Here's how the part is built. I have some questions about the finished solid (model axes, mm). A direction names the side the tool comes from. Round coordinates to 2 decimals unless told otherwise and drop trailing zeros. Loops run counter-clockwise (first coordinate to the right, second up) from the corner with the lowest first, then second, coordinate; pieces in that order, holes last. Notation, with made-up numbers: M 34,54.5 L 77,54.5 A16 cw 77,65.5 Z; hole C 21,21 d4. An arc over 180 degrees is marked long. Answer as CSV lines item,"result".
```python
from build123d import *

# Parameters (mm, degrees)
SKETCH_1_R               = 12.5
EXTRUDE_1_DEPTH          = 7.5
EXTRUDE_2_DEPTH          = 10
EXTRUDE_START            = -4.5
SKETCH_3_R               = 18
SKETCH_3_R_2             = 12.5
EXTRUDE_3_DEPTH          = 4.5
SKETCH_4_R               = 2.1
CUT_EXTRUDE_1_DEPTH      = 39.055354
SKETCH_5_R               = 1.6
CUT_EXTRUDE_2_DEPTH      = 39.055354
CUT_EXTRUDE_START        = -10
CUT_EXTRUDE_3_DEPTH      = 10
SKETCH_7_R               = 21
EXTRUDE_4_DEPTH          = 3
SKETCH_8_R               = 1.6
CUT_EXTRUDE_4_DEPTH      = 41.816663
SKETCH_13_R              = 15
SKETCH_13_R_2            = 12.5
EXTRUDE_6_DEPTH          = 10.5
CUT_EXTRUDE_6_DEPTH      = 39.820098
CUT_EXTRUDE_6_DEPTH_BACK = 39.820098
CUT_EXTRUDE_START_2      = 10.5
SKETCH_9_R               = 3.4
CUT_EXTRUDE_5_DEPTH      = 15
EXTRUDE_5_DEPTH          = 10
SKETCH_12_R              = 1.6
CUT_EXTRUDE_7_DEPTH      = 47.859471


# Read off the part's stored shape, not the designer's step: 凸台-拉伸2
with BuildPart() as part:
    # 草图1 → 凸台-拉伸1 (new, symmetric)
    with BuildSketch(Plane(origin=(0, 0, 0), x_dir=(1, 0, 0), z_dir=(0, 1, 0))):
        with Locations(Location((0, 0, 0), (0, 0, 270))):
            Circle(SKETCH_1_R)
        with BuildLine():
            Line((6.6, -7.6), (-6.6, -7.6))
            ThreePointArc((-6.6, -7.6), (-8.307107, -8.307107), (-7.6, -6.6))
            Line((-7.6, -6.6), (-7.6, 6.6))
            ThreePointArc((-7.6, 6.6), (-8.307107, 8.307107), (-6.6, 7.6))
            Line((-6.6, 7.6), (6.6, 7.6))
            ThreePointArc((6.6, 7.6), (7.6, 8.6), (8.6, 7.6))
            ThreePointArc((8.6, 7.6), (8.307107, 6.892893), (7.6, 6.6))
            Line((7.6, 6.6), (7.6, -6.6))
            ThreePointArc((7.6, -6.6), (8.307107, -6.892893), (8.6, -7.6))
            ThreePointArc((8.6, -7.6), (7.6, -8.6), (6.6, -7.6))
        make_face(mode=Mode.SUBTRACT)
    extrude(amount=EXTRUDE_1_DEPTH, both=True)

    # 凸台-拉伸2 outline → 凸台-拉伸2 (add)
    with BuildSketch(Plane.XZ.offset(7.5)):
        with BuildLine():
            Line((10.6, -6.624953), (10.6, 6.624953))
            ThreePointArc((10.6, 6.624953), (8.838835, 8.838835), (6.624953, 10.6))
            Line((6.624953, 10.6), (-6.624953, 10.6))
            ThreePointArc((-6.624953, 10.6), (-8.838835, 8.838835), (-10.6, 6.624953))
            Line((-10.6, 6.624953), (-10.6, -6.624953))
            ThreePointArc((-10.6, -6.624953), (-8.838835, -8.838835), (-6.624953, -10.6))
            Line((-6.624953, -10.6), (6.624953, -10.6))
            ThreePointArc((6.624953, -10.6), (8.838835, -8.838835), (10.6, -6.624953))
        make_face()
        with BuildLine():
            ThreePointArc((-6.6, -7.6), (-8.307107, -8.307107), (-7.6, -6.6))
            Line((-7.6, -6.6), (-7.6, 6.6))
            ThreePointArc((-7.6, 6.6), (-8.307107, 8.307107), (-6.6, 7.6))
            Line((-6.6, 7.6), (6.6, 7.6))
            ThreePointArc((6.6, 7.6), (8.307107, 8.307107), (7.6, 6.6))
            Line((7.6, 6.6), (7.6, -6.6))
            ThreePointArc((7.6, -6.6), (8.307107, -8.307107), (6.6, -7.6))
            Line((6.6, -7.6), (-6.6, -7.6))
        make_face(mode=Mode.SUBTRACT)
    extrude_2 = extrude(amount=EXTRUDE_2_DEPTH)

    # 镜向1: 凸台-拉伸2 across plane
    add(extrude_2.mirror(Plane.ZX))

    # 草图3 → 凸台-拉伸3 (add)
    with BuildSketch(Plane.XZ.offset(7.5).offset(EXTRUDE_START)):
        with Locations(Location((0, 0, 0), (0, 0, 270))):
            Circle(SKETCH_3_R)
        with Locations(Location((0, 0, 0), (0, 0, 270))):
            Circle(SKETCH_3_R_2, mode=Mode.SUBTRACT)
    extrude(amount=EXTRUDE_3_DEPTH)

    # 草图4 → 切除-拉伸1 (cut, through all)
    with BuildSketch(Plane.XY.offset(10.6)):
        with Locations((0, -12.5)):
            Circle(SKETCH_4_R)
    extrude(amount=-CUT_EXTRUDE_1_DEPTH, mode=Mode.SUBTRACT)

    # 草图5 → 切除-拉伸2 (cut, through all)
    with BuildSketch(Plane(origin=(10.6, 0, 0), x_dir=(0, 0, -1), z_dir=(1, 0, 0))):
        with Locations((0, 12.5)):
            Circle(SKETCH_5_R)
    extrude(amount=-CUT_EXTRUDE_2_DEPTH, mode=Mode.SUBTRACT)

    # 草图6 → 切除-拉伸3 (cut)
    with BuildSketch(Plane.XZ.offset(17.5).offset(CUT_EXTRUDE_START)):
        with BuildLine():
            Line((10.6, -6.624953), (10.6, 6.624953))
            ThreePointArc((10.6, 6.624953), (8.838835, 8.838835), (6.624953, 10.6))
            Line((6.624953, 10.6), (-6.624953, 10.6))
            ThreePointArc((-6.624953, 10.6), (-8.838835, 8.838835), (-10.6, 6.624953))
            Line((-10.6, 6.624953), (-10.6, -6.624953))
            ThreePointArc((-10.6, -6.624953), (-8.838835, -8.838835), (-6.624953, -10.6))
            Line((-6.624953, -10.6), (6.624953, -10.6))
            ThreePointArc((6.624953, -10.6), (8.838835, -8.838835), (10.6, -6.624953))
        make_face()
    extrude(amount=CUT_EXTRUDE_3_DEPTH, mode=Mode.SUBTRACT)

    # 草图7 → 凸台-拉伸4 (add)
    with BuildSketch(Plane.XZ.offset(7.5)):
        with Locations(Location((0, 0, 0), (0, 0, 270))):
            Circle(SKETCH_7_R)
    extrude(amount=EXTRUDE_4_DEPTH)

    # 草图8 → 切除-拉伸4 (cut, through all)
    with BuildSketch(Plane.XZ.offset(10.5)):
        with Locations(Location((0, 16, 0), (0, 0, 270))):
            Circle(SKETCH_8_R)
        with Locations(Location((16, 0, 0), (0, 0, 270))):
            Circle(SKETCH_8_R)
        with Locations(Location((0, -16, 0), (0, 0, 270))):
            Circle(SKETCH_8_R)
        with Locations(Location((-16, 0, 0), (0, 0, 270))):
            Circle(SKETCH_8_R)
    extrude(amount=-CUT_EXTRUDE_4_DEPTH, mode=Mode.SUBTRACT)

    # 草图13 → 凸台-拉伸6 (add)
    with BuildSketch(Plane(origin=(0, -3, 0), x_dir=(1, 0, 0), z_dir=(0, 1, 0))):
        with Locations(Location((0, 0, 0), (0, 0, 85.379415))):
            Circle(SKETCH_13_R)
        Circle(SKETCH_13_R_2, mode=Mode.SUBTRACT)
    extrude(amount=EXTRUDE_6_DEPTH)

    # 草图10 → 切除-拉伸6 (cut, two sides: drawn at the far end of the back side and taken through both)
    with BuildSketch(Plane(origin=(0, -7.5, 0), x_dir=(1, 0, 0), z_dir=(0, 1, 0)).offset(-CUT_EXTRUDE_6_DEPTH_BACK)):
        with BuildLine():
            Line((-7.6, 6.6), (-7.6, -6.6))
            ThreePointArc((-7.6, -6.6), (-8.307107, -8.307107), (-6.6, -7.6))
            Line((-6.6, -7.6), (6.6, -7.6))
            ThreePointArc((6.6, -7.6), (8.307107, -8.307107), (7.6, -6.6))
            Line((7.6, -6.6), (7.6, 6.6))
            ThreePointArc((7.6, 6.6), (8.307107, 8.307107), (6.6, 7.6))
            Line((6.6, 7.6), (-6.6, 7.6))
            ThreePointArc((-6.6, 7.6), (-8.307107, 8.307107), (-7.6, 6.6))
        make_face()
    extrude(amount=CUT_EXTRUDE_6_DEPTH + CUT_EXTRUDE_6_DEPTH_BACK, mode=Mode.SUBTRACT)

    # 草图9 → 切除-拉伸5 (cut)
    with BuildSketch(Plane(origin=(0, -3, 0), x_dir=(1, 0, 0), z_dir=(0, 1, 0)).offset(CUT_EXTRUDE_START_2)):
        with Locations((0, -16)):
            Circle(SKETCH_9_R)
        with Locations((16, 0)):
            Circle(SKETCH_9_R)
        with Locations((0, 16)):
            Circle(SKETCH_9_R)
        with Locations((-16, 0)):
            Circle(SKETCH_9_R)
    extrude(amount=-CUT_EXTRUDE_5_DEPTH, mode=Mode.SUBTRACT)

    # 草图11 → 凸台-拉伸5 (add)
    with BuildSketch(Plane(origin=(0, 17.5, 0), x_dir=(1, 0, 0), z_dir=(0, 1, 0))):
        with BuildLine():
            Line((6.624953, 10.6), (-6.624953, 10.6))
            ThreePointArc((-6.624953, 10.6), (-8.838835, 8.838835), (-10.6, 6.624953))
            Line((-10.6, 6.624953), (-10.6, -6.624953))
            ThreePointArc((-10.6, -6.624953), (-8.838835, -8.838835), (-6.624953, -10.6))
            Line((-6.624953, -10.6), (6.624953, -10.6))
            ThreePointArc((6.624953, -10.6), (8.838835, -8.838835), (10.6, -6.624953))
            Line((10.6, -6.624953), (10.6, 6.624953))
            ThreePointArc((10.6, 6.624953), (8.838835, 8.838835), (6.624953, 10.6))
        make_face()
        with BuildLine():
            Line((-6.6, -7.6), (6.6, -7.6))
            ThreePointArc((6.6, -7.6), (8.307107, -8.307107), (7.6, -6.6))
            Line((7.6, -6.6), (7.6, 6.6))
            ThreePointArc((7.6, 6.6), (8.307107, 8.307107), (6.6, 7.6))
            Line((6.6, 7.6), (-6.6, 7.6))
            ThreePointArc((-6.6, 7.6), (-8.307107, 8.307107), (-7.6, 6.6))
            Line((-7.6, 6.6), (-7.6, -6.6))
            ThreePointArc((-7.6, -6.6), (-8.307107, -8.307107), (-6.6, -7.6))
        make_face(mode=Mode.SUBTRACT)
    extrude(amount=EXTRUDE_5_DEPTH)

    # 草图12 → 切除-拉伸7 (cut, through all)
    with BuildSketch(Plane(origin=(0, 0, -10.6), x_dir=(-1, 0, 0), z_dir=(0, 0, -1))):
        with Locations((0, 22.5)):
            Circle(SKETCH_12_R)
    extrude(amount=-CUT_EXTRUDE_7_DEPTH, mode=Mode.SUBTRACT)


solid = part.part
```
1. If I drill on line 1 (Y direction, x = -9, z = 0); line 2 (Y direction, x = -8.5, z = 18); line 3 (Z direction, x = 2, y = 20), over which ranges is the centre line in solid material (lowest first)? Write a range as [from, to].
Evaluation:
line 1,"y = [-10.5, 10.9], [14.1, 27.5]"
line 2,"y = [-10.5, -7.5]"
line 3,"z = [-10.6, -7.6], [7.6, 10.6]"
2. I want a section at D-D, the plane x = -6. Please give me the cut outline in (y, z).
Evaluation:
outline,"M -10.5,-20.12 L -7.5,-20.12 L -7.5,-16.97 L -3,-16.97 L -3,-13.75 L 7.5,-13.75 L 7.5,-10.6 L 27.5,-10.6 L 27.5,-7.6 L -10.5,-7.6 Z; M -10.5,7.6 L 27.5,7.6 L 27.5,10.6 L 7.5,10.6 L 7.5,13.75 L -3,13.75 L -3,16.97 L -7.5,16.97 L -7.5,20.12 L -10.5,20.12 Z"
3. Which directions (+Z, -Z, +X, -X, +Y, -Y) give clear straight access to the entire face, cutting with the end or side of a thin tool? Please do faces 1 (the flat face through (10.6, 17, 0)), 2 (the flat face through (-11, -3, -11)), 3 (the flat face through (11, -3, -11)).
Evaluation:
face 1,"+Z, -Z, +X, +Y"
face 2,"-Z, -X, +Y"
face 3,"-Z, +X, +Y"
4. I want a section at B-B, the plane y = 22.5. Please give me the cut outline in (x, z).
Evaluation:
outline,"M -10.6,-6.62 A12.5 ccw -6.62,-10.6 L -1.6,-10.6 L -1.6,-7.6 L -6.6,-7.6 A1 cw long -7.6,-6.6 L -7.6,6.6 A1 cw long -6.6,7.6 L -1.6,7.6 L -1.6,10.6 L -6.62,10.6 A12.5 ccw -10.6,6.62 Z; M 1.6,-10.6 L 6.62,-10.6 A12.5 ccw 10.6,-6.62 L 10.6,6.62 A12.5 ccw 6.62,10.6 L 1.6,10.6 L 1.6,7.6 L 6.6,7.6 A1 cw long 7.6,6.6 L 7.6,-6.6 A1 cw long 6.6,-7.6 L 1.6,-7.6 Z"
5. I want a section at A-A, the plane y = -6. Please give me the cut outline in (x, z), and give its area (3 significant figures).
Evaluation:
outline,"M -17.76,-2.91 A18 ccw -2.91,-17.76 A3.4 cw long 2.91,-17.76 A18 ccw 17.76,-2.91 A3.4 cw long 17.76,2.91 A18 ccw 2.91,17.76 A3.4 cw long -2.91,17.76 A18 ccw -17.76,2.91 A3.4 cw long Z; hole M -7.6,-6.6 A1 ccw long -6.6,-7.6 L 6.6,-7.6 A1 ccw long 7.6,-6.6 L 7.6,6.6 A1 ccw long 6.6,7.6 L -6.6,7.6 A1 ccw long -7.6,6.6 Z"
area,"655 mm²"
6. For P1, Ø1.5, axis at y = 0, z = 9.5, coming from the +X side; P2, Ø1.8, axis at x = -7.6, z = 7.6, coming from the +Y side; P3, Ø4, axis at y = 12.5, z = 0, coming from the -X side; P4, Ø4, axis at y = 14.5, z = 0, coming from the +X side, each with a flat end and sliding along its axis, tell me the tip position at first contact or that it passes through.
Evaluation:
P1,"stops at x = 12.18"
P2,"passes through"
P3,"stops at x = -10.6"
P4,"stops at x = 10.6"
7. We'd pull the mould along X, two halves only. Please class faces 4 (the cylindrical face through (8.81, 17.36, 8.87)), 5 (the flat face through (11, -3, 11)), 6 (the flat face through (-7.6, 8, 0)): pulls with the +X half, pulls with the -X half, needs draft (parallel to the pull), parting line crosses it, or undercut.
Evaluation:
face 4,"pulls with the +X half"
face 5,"needs draft"
face 6,"undercut"
8. I want a section at C-C, the plane z = 4.5. Please give me the cut outline in (x, y), and give its area (3 significant figures).
Evaluation:
outline,"M -20.51,-10.5 L -7.6,-10.5 L -7.6,27.5 L -10.6,27.5 L -10.6,7.5 L -14.31,7.5 L -14.31,-3 L -17.43,-3 L -17.43,-7.5 L -20.51,-7.5 Z; M 7.6,-10.5 L 20.51,-10.5 L 20.51,-7.5 L 17.43,-7.5 L 17.43,-3 L 14.31,-3 L 14.31,7.5 L 10.6,7.5 L 10.6,27.5 L 7.6,27.5 Z"
area,"427 mm²"
